Could you check a few things on this model? Use its own coordinates, in mm. A direction names the side the tool comes from. Coordinates: 2 decimals unless noted, no trailing zeros. Write each loop counter-clockwise with the first axis right and the second up, starting at its lowest first coordinate (ties: lowest second). Pieces come first, ordered by that corner, then holes.
```python
from build123d import *

# Parameters (mm, degrees)
BOSS_EXTRUDE2_DEPTH = 90
BOSS_EXTRUDE3_DEPTH = 12
SKETCH3_W           = 18
SKETCH3_H           = 76.981608939
SKETCH3_W_2         = 12
SKETCH3_H_2         = 76.255384777
BOSS_EXTRUDE4_DEPTH = 60
BOSS_EXTRUDE5_START = -250
BOSS_EXTRUDE5_DEPTH = 250
SKETCH5_R           = 10
BOSS_EXTRUDE6_DEPTH = 160
SKETCH8_R           = 10


with BuildPart() as part:
    # Sketch1 → Boss-Extrude2 (new, symmetric)
    with BuildSketch(Plane.XY):
        with BuildLine():
            Line((0, 0), (0, 220))
            ThreePointArc((0, 220), (45.729180399, 144.95403091), (59.974042828, 58.235294118))
            ThreePointArc((59.974042828, 58.235294118), (41.797832761, 16.954196761), (0, 0))
        make_face()
    extrude(amount=BOSS_EXTRUDE2_DEPTH, both=True)

    # Sketch2 → Boss-Extrude3 (add)
    with BuildSketch(Plane.ZY):
        Polygon((0, 0), (125, 0), (125, 270), (-125, 270), (-125, 0), align=None)
    extrude(amount=BOSS_EXTRUDE3_DEPTH)

    # Sketch3 → Boss-Extrude4 (add, symmetric)
    with BuildSketch(Plane.XY):
        with Locations((26, 161.50919553)):
            Rectangle(SKETCH3_W, SKETCH3_H)
        with Locations((6, 211.872307612)):
            Rectangle(SKETCH3_W_2, SKETCH3_H_2)
    extrude(amount=BOSS_EXTRUDE4_DEPTH, both=True)

    # Sketch4 → Boss-Extrude5 (add)
    with BuildSketch(Plane.XY.offset(125).offset(BOSS_EXTRUDE5_START)):
        with BuildLine():
            Line((0, 65), (25, 65))
            ThreePointArc((25, 65), (45, 45), (25, 25))
            Line((25, 25), (0, 25))
            Line((0, 25), (0, 65))
        make_face()
        with BuildLine():
            Line((0, 205), (0, 175))
            ThreePointArc((0, 175), (15, 190), (0, 205))
        make_face()
    extrude(amount=BOSS_EXTRUDE5_DEPTH)

    # Sketch5 → Boss-Extrude6 (add)
    with BuildSketch(Plane(origin=(0, 0, 0), x_dir=(0, 0, -1), z_dir=(1, 0, 0))):
        with Locations((0, 58.235294118)):
            Circle(SKETCH5_R)
    extrude(amount=BOSS_EXTRUDE6_DEPTH)

    # Sketch6 → Revolve2 (revolve)
    with BuildSketch(Plane(origin=(0, 58, 0), x_dir=(1, 0, 0), z_dir=(0, 1, 0))):
        with BuildLine():
            Line((81.674631605, 0), (101.674631605, 0))
            ThreePointArc((101.674631605, 0), (96.000878794, 12.625507314), (82.792800006, 16.765744099))
            Line((82.792800006, 16.765744099), (79.883742711, 13.856686803))
            ThreePointArc((79.883742711, 13.856686803), (73.043114259, 18.427448605), (64.974042828, 20.032486705))
            Line((64.974042828, 20.032486705), (64.974042828, 0))
            Line((64.974042828, 0), (81.674631605, 0))
        make_face()
    revolve(axis=Axis((64.974042828, 58, 0), (1, 0, 0)))

    # Sweep1: sweep along a path in Sketch7
    with BuildLine(Plane.XY) as sweep1_path:
        Line((160, 58.235294118), (329.144671741, 119.798919916))
    # Sketch8 → Sweep1 (sweep)
    with BuildSketch(Plane(origin=(160, 0, 0), x_dir=(0, 0, -1), z_dir=(1, 0, 0))):
        with Locations((0, 58.235294118)):
            Circle(SKETCH8_R)
    sweep(path=sweep1_path.line)

    # Sketch9 → Revolve3 (revolve)
    with BuildSketch(Plane.XY):
        with BuildLine():
            Line((329.144671741, 119.798919916), (329.144671741, 79.798919916))
            ThreePointArc((329.144671741, 79.798919916), (369.144671741, 119.798919916), (329.144671741, 159.798919916))
            Line((329.144671741, 159.798919916), (329.144671741, 119.798919916))
        make_face()
    revolve(axis=Axis((329.144671741, 119.798919916, 0), (0, -1, 0)))


solid = part.part
```
Item 1: I want a section at D-D, the plane x = 145. List the corners of the cut face in (y, z) for me, then the cut area to 3 significant figures.
Item 2: Which directions (+Z, -Z, +X, -X, +Y, -Y) give clear straight access to the entire face, cutting with the end or side of a thin tool? Please do faces 1 (the flat face through (12, 228, 1)), 2 (the flat face through (6, 233, -60)), 3 (the cylindrical face through (15, 190, -108)), 4 (the flat face through (0, 13, -108)).
Item 3: Will these pins go through, and if not, where does the flat tip stop? pin 1 Ø9 at (x, y) = (22, 190) entering from +Z; pin 2 Ø20 at (y, z) = (12.5, 114) entering from +X; pin 3 Ø24.5 at (y, z) = (178, -2.5) entering from +X.
Item 4: If I drill on line 1 along X through (y, z) = (217.5, -27.5); line 2 along X through (y, z) = (185.5, -39); line 3 along X through (y, z) = (199.5, -57.5), over which ranges is the centre line in solid material (lowest first)?
Item 5: I want a section at B-B, the plane z = 55.5. List the corners of the cut face in (x, y) for me.
Item 6: If we mould it in two halves opening along Y, with no side actions, what happens to faces 5 (the flat face through (-6, 0, -2)), 6 (the flat face through (24, 112, -90)), 7 (the flat face through (28, 192, -60)), 8 (the cylindrical face through (45, 45, 107))? For each: released by +Y, released by -Y, zero draft, split by the parting line, or undercut.
Item 7: I want a section at A-A, the plane z = -28. List the corners of the cut face in (x, y) for me, then the cut area to 3 significant figures.
Item 8: I want a section at C-C, the plane y = 190. List the corners of the cut face in (x, z) for me.
Taken from the geometry:
1. outline: circle Ø20 at (58.24, 0)
1. area: 314 mm2
2. face 1: +Z, -Z, +X, +Y
2. face 2: -Z, +X, +Y
2. face 3: -Z, +X
2. face 4: -Z, +X, -Y
3. pin 1: stops at z = 90
3. pin 2: stops at x = 0
3. pin 3: stops at x = 36.83
4. line 1: x = -12 to 12
4. line 2: x = -12 to 35
4. line 3: x = -12 to 16.65, 17 to 35
5. outline: (-12, 0) - (0, 0) arc R60 ccw to (59.97, 58.24) arc R230 ccw to (35, 169.43) - (35, 200) - (17, 200) - (17, 199.01) arc R230 ccw to (12, 205.72) - (12, 250) - (0, 250) - (0, 270) - (-12, 270) - close
6. face 5: released by -Y
6. face 6: undercut
6. face 7: zero draft
6. face 8: split by the parting line
7. outline: (-12, 0) - (0, 0) arc R60 ccw to (59.97, 58.24) arc R230 ccw to (35, 169.43) - (35, 200) - (17, 200) - (17, 199.01) arc R230 ccw to (12, 205.72) - (12, 250) - (0, 250) - (0, 270) - (-12, 270) - close; circle Ø57.13 at (329.14, 119.8)
7. area: 16,000 mm2
8. outline: (-12, -125) - (15, -125) - (15, -90) - (23.14, -90) - (23.14, -60) - (35, -60) - (35, 60) - (23.14, 60) - (23.14, 90) - (15, 90) - (15, 125) - (-12, 125) - close
